Can you work these out from the model? Positions are in its coordinate system, mm. A direction names the side the tool comes from. Coordinates: 2 decimals unless noted, no trailing zeros. Loops run counter-clockwise (first coordinate to the right, second up) from the corner with the lowest first, then second, coordinate; pieces in that order, holes last.
```python
from build123d import *

# Parameters (mm, degrees)
EXTRUDE_START   = -6
EXTRUDE_1_DEPTH = 14.374594
SKETCH_3_R      = 34
EXTRUDE_2_DEPTH = 8
SKETCH_5_R      = 18
EXTRUDE_3_DEPTH = 6.5


with BuildPart() as part:
    # Эскиз1 → Вытянуть1 (new body)
    with BuildSketch(Plane.XY.offset(EXTRUDE_START)):
        with BuildLine():
            ThreePointArc((-2.5, 17.82554347), (-15.588457268, 9), (-16.687373481, -6.747708226))
            ThreePointArc((-16.687373481, -6.747708226), (-14.029608141, -8.099998037), (-14.187373481, -11.077835244))
            ThreePointArc((-14.187373481, -11.077835244), (0, -18), (14.187373481, -11.077835244))
            ThreePointArc((14.187373481, -11.077835244), (14.029608141, -8.099998037), (16.687373481, -6.747708226))
            ThreePointArc((16.687373481, -6.747708226), (15.588457268, 9), (2.5, 17.82554347))
            ThreePointArc((2.5, 17.82554347), (0, 16.199996074), (-2.5, 17.82554347))
        make_face()
        with BuildLine():
            Line((-2, 8.85), (2, 8.85))
            Line((2, 8.85), (2, 6.708203932))
            ThreePointArc((2, 6.708203932), (0, -7), (-2, 6.708203932))
            Line((-2, 6.708203932), (-2, 8.85))
        make_face(mode=Mode.SUBTRACT)
    extrude(amount=EXTRUDE_1_DEPTH)

    # Эскиз3 → Вытянуть2 (add)
    with BuildSketch(Plane.XY.offset(8.374593773)):
        Circle(SKETCH_3_R)
        with BuildLine():
            Line((-2, 8.85), (-2, 6.708203932))
            ThreePointArc((-2, 6.708203932), (0, -7), (2, 6.708203932))
            Line((2, 6.708203932), (2, 8.85))
            Line((2, 8.85), (-2, 8.85))
        make_face(mode=Mode.SUBTRACT)
    extrude(amount=EXTRUDE_2_DEPTH)

    # Эскиз5 → Вытянуть3 (add)
    with BuildSketch(Plane.XY.offset(16.374593773)):
        with Locations(Location((0, 0, 0), (0, 0, 180))):
            Circle(SKETCH_5_R)
        with BuildLine():
            Line((-2, 6.708203932), (-2, 8.85))
            Line((-2, 8.85), (2, 8.85))
            Line((2, 8.85), (2, 6.708203932))
            ThreePointArc((2, 6.708203932), (0, -7), (-2, 6.708203932))
        make_face(mode=Mode.SUBTRACT)
    extrude(amount=EXTRUDE_3_DEPTH)


solid = part.part
```
Item 1: Suppose I cut it at D-D, the plane x = -10. Please give me the cut outline in (y, z), plus the area to 3 significant figures.
Results are:
outline: (-32.5, 8.37) - (-14.97, 8.37) - (-14.97, -6) - (14.97, -6) - (14.97, 8.37) - (32.5, 8.37) - (32.5, 16.37) - (14.97, 16.37) - (14.97, 22.87) - (-14.97, 22.87) - (-14.97, 16.37) - (-32.5, 16.37) - close
area: 1,140 mm2
Item 2: On a 3-axis mill with a long thin cutter (end or side, diameter ignored), from which of +Z, -Z, +X, -X, +Y, -Y can I reach the whole of each face in a straight line? I mean faces 1 (the face through (15.7, 8.8, 1.1)), 2 (the face through (-15.47, 9.2, 1.09)), 3 (the face through (0, -18, 1)), 4 (the face through (-16, -7, 8.375)). Say none if no direction works.
Results are:
face 1: -Z, +X
face 2: -Z, -X
face 3: -Z, -Y
face 4: -Z
Item 3: We'd pull the mould along Y, two halves only. Please class faces 5 (the face through (-14.052, -8.062, 1.087)), 6 (the face through (13.267, -12.165, 19.579)), 7 (the face through (15, -15, 16.375)): +Y half, -Y half, draft (parallel to the pull), parting line (faces both ways), or undercut.
Results are:
face 5: undercut
face 6: parting line
face 7: draft
Item 4: I need wall thicknesses on line 1 along X through (y, z) = (0, 1.75); line 2 along Y through (x, z) = (0, 10.5); line 3 along Y through (x, z) = (0, 18.25). Which ranges of each line are inside material? Lowest first, please.
Results are:
line 1: x = -18 to -7, 7 to 18
line 2: y = -34 to -7, 8.85 to 34
line 3: y = -18 to -7, 8.85 to 18
Item 5: Suppose I cut it at B-B, the plane x = 0. Please give me the cut outline in (y, z).
Results are:
outline: (-34, 8.37) - (-18, 8.37) - (-18, -6) - (-7, -6) - (-7, 22.87) - (-18, 22.87) - (-18, 16.37) - (-34, 16.37) - close; (8.85, -6) - (16.2, -6) - (16.2, 8.37) - (34, 8.37) - (34, 16.37) - (18, 16.37) - (18, 22.87) - (8.85, 22.87) - close
Item 6: Suppose I cut it at A-A, the plane y = 0. Please give me the cut outline in (x, z), plus the area to 3 significant figures.
Results are:
outline: (-34, 8.37) - (-18, 8.37) - (-18, -6) - (-7, -6) - (-7, 22.87) - (-18, 22.87) - (-18, 16.37) - (-34, 16.37) - close; (7, -6) - (18, -6) - (18, 8.37) - (34, 8.37) - (34, 16.37) - (18, 16.37) - (18, 22.87) - (7, 22.87) - close
area: 891 mm2
Item 7: Suppose I cut it at C-C, the plane z = 4.75. Please give me the cut outline in (x, y), plus the area to 3 significant figures.
Results are:
outline: (-16.69, -6.75) arc R2.74 cw to (-14.19, -11.08) arc R18 ccw to (14.19, -11.08) arc R2.74 cw to (16.69, -6.75) arc R18 ccw to (2.5, 17.83) arc R2.74 cw to (-2.5, 17.83) arc R18 ccw to start; hole (-2, 6.71) arc R7 ccw (long way) to (2, 6.71) - (2, 8.85) - (-2, 8.85) - close
area: 837 mm2
Item 8: I'm going to push flat-ended pins straight in: P1, Ø2.5, axis at y = 8, z = 9.5, coming from the +X side; P2, Ø12, axis at y = -24, z = 14.5, coming from the -X side; P3, Ø6, axis at y = -14, z = 19, coming from the +X side; P4, Ø1.5, axis at x = 3.5, y = 4.5, coming from the -Z side. Where does each tip first touch, or does it pass through?
Results are:
P1: stops at x = 33.32
P2: stops at x = -28.84
P3: stops at x = 31.6
P4: passes through
